Source: CAD feature listing. Evaluate the final solid. Frame: model axes, mm. Face numbers are marked on the shaded views. A direction names the side the tool comes from. Give positions to 0.01 mm unless a question says otherwise; leave off trailing zeros. Order: outer loops, then holes, each group sorted by start corner. A loop starts at its lowest first (then second) coordinate and runs counter-clockwise, first axis right, second up.
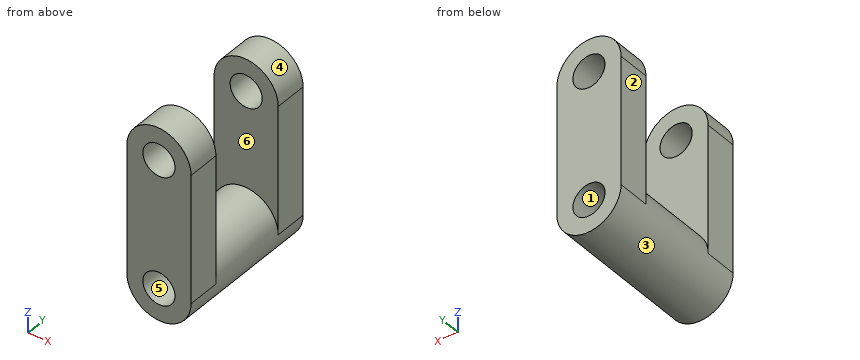
from build123d import *
from build123d import SkipClean  # not in build123d's __all__

# Parameters (mm, degrees)
F0_R     = 12.7
F1_DEPTH = 25.4
F2_R     = 25.4
F2_R_2   = 12.4458783194
F3_DEPTH = 63.5
F4_R     = 12.7
F5_DEPTH = 25.4


# Not quite as in the source:
# - after a boolean that leaves OpenCascade's solid faulty, fix() repairs it


with BuildPart() as f1:
    # F0 (on Front) → F1 (new body)
    with BuildSketch(Plane.XZ):
        with BuildLine():
            ThreePointArc((-25.4, -50.8), (0, -76.2), (25.4, -50.8))
            Line((25.4, -50.8), (25.4, 50.8))
            ThreePointArc((25.4, 50.8), (0, 76.2), (-25.4, 50.8))
            Line((-25.4, 50.8), (-25.4, -50.8))
        make_face()
        with Locations((0, -50.8)):
            Circle(F0_R, mode=Mode.SUBTRACT)
        with Locations((0, 50.8)):
            Circle(F0_R, mode=Mode.SUBTRACT)
    extrude(amount=-F1_DEPTH)

    # F2 (on face) → F3 (join)
    with BuildSketch(Plane.XZ):
        with Locations((0, -50.8)):
            Circle(F2_R)
        with Locations((0, -50.8)):
            Circle(F2_R_2, mode=Mode.SUBTRACT)
    with SkipClean():  # cleaning this boolean's faces spoils the solid; the shape is the same uncleaned
        extrude(amount=F3_DEPTH)

    # F4 (on face) → F5 (join)
    with BuildSketch(Plane.XZ.offset(63.5)):
        with BuildLine():
            Line((-25.4, 50.8), (-25.4, -50.8))
            ThreePointArc((-25.4, -50.8), (0, -25.4), (25.4, -50.8))
            Line((25.4, -50.8), (25.4, 50.8))
            ThreePointArc((25.4, 50.8), (0, 76.2), (-25.4, 50.8))
        make_face()
        with Locations((0, 50.8)):
            Circle(F4_R, mode=Mode.SUBTRACT)
        with BuildLine():
            ThreePointArc((25.4, -50.8), (0, -25.4), (-25.4, -50.8))
            ThreePointArc((-25.4, -50.8), (0, -76.2), (25.4, -50.8))
        make_face()
        with Locations((0, -50.8)):
            Circle(F4_R, mode=Mode.SUBTRACT)
    extrude(amount=F5_DEPTH)

    add(f1.part.fix(), mode=Mode.REPLACE)


solid = f1.part
1) Pull-direction query (Z, two-part tool) for the marked faces 4, 5 and 6; classes: +Z half, -Z half, draft (parallel to the pull), parting line (faces both ways), or undercut.
Checks:
face 4: +Z half
face 5: undercut
face 6: draft
2) Section query B-B on z = 21.5. Output: boundary loops of the cut face in (x, y), and give its area (3 significant figures).
Checks:
outline: (-25.4, -88.9) - (25.4, -88.9) - (25.4, -63.5) - (-25.4, -63.5) - close; (-25.4, 0) - (25.4, 0) - (25.4, 25.4) - (-25.4, 25.4) - close
area: 2,580 mm2
3) Ray query, L1, parallel to Z at x = 0, y = -74; L2, parallel to Y at x = 0.5, z = 3; L3, parallel to Z at x = 0, y = -55. Return the intervals inside material, ascending.
Checks:
L1: z = -76.2 to -63.5, -38.1 to 38.1, 63.5 to 76.2
L2: y = -88.9 to -63.5, 0 to 25.4
L3: z = -76.2 to -63.25, -38.35 to -25.4
4) Section query D-D on x = -15.5. Output: boundary loops of the cut face in (y, z).
Checks:
outline: (-88.9, -70.92) - (25.4, -70.92) - (25.4, 70.92) - (0, 70.92) - (0, -30.68) - (-63.5, -30.68) - (-63.5, 70.92) - (-88.9, 70.92) - close
5) Reachability of the marked faces 1, 2 and 3 from +Z, -Z, +X, -X, +Y, -Y: full face, straight path, thin tool, end or side. Return the list, or none.
Checks:
face 1: +Y
face 2: +Z, -Z, -X, +Y, -Y
face 3: none
6) Section query A-A on x = 0. Output: boundary loops of the cut face in (y, z).
Checks:
outline: (-88.9, -76.2) - (25.4, -76.2) - (25.4, -63.5) - (0, -63.5) - (0, -63.25) - (-63.5, -63.25) - (-63.5, -63.5) - (-88.9, -63.5) - close; (-88.9, -38.1) - (-63.5, -38.1) - (-63.5, -38.35) - (0, -38.35) - (0, -38.1) - (25.4, -38.1) - (25.4, 38.1) - (0, 38.1) - (0, -25.4) - (-63.5, -25.4) - (-63.5, 38.1) - (-88.9, 38.1) - close; (-88.9, 63.5) - (-63.5, 63.5) - (-63.5, 76.2) - (-88.9, 76.2) - close; (0, 63.5) - (25.4, 63.5) - (25.4, 76.2) - (0, 76.2) - close
7) First-contact query: pin 1 Ø10 at (x, y) = (-2, -5.5) entering from -Z; pin 2 Ø23 at (x, z) = (0, -50.8) entering from +Y; pin 3 Ø5 at (x, y) = (19, -7.5) entering from -Z; pin 4 Ø1.5 at (x, y) = (12, -21.5) entering from -Z. Flat tips, straight axial feed; report the tip coordinate or a pass-through.
Checks:
pin 1: stops at z = -76.2
pin 2: passes through
pin 3: stops at z = -70.11
pin 4: stops at z = -73.57
8) Section query C-C on y = 14. Output: boundary loops of the cut face in (x, z), and give its area (3 significant figures).
Checks:
outline: (-25.4, -50.8) arc R25.4 ccw to (25.4, -50.8) - (25.4, 50.8) arc R25.4 ccw to (-25.4, 50.8) - close; hole circle Ø25.4 at (0, -50.8); hole circle Ø25.4 at (0, 50.8)
area: 6,170 mm2
